```python
from build123d import *

# Parameters (mm, degrees)
SKETCH002_R     = 6
SKETCH002_R_2   = 3
SKETCH002_R_3   = 1.25
SKETCH002_R_4   = 2
SKETCH002_R_5   = 12
PAD_DEPTH       = 28.575
POCKET_DEPTH    = 16.075
SKETCH_R        = 13.05
POCKET001_DEPTH = 10
SKETCH005_R     = 13.05
POCKET002_DEPTH = 10
SKETCH006_R     = 3
POCKET003_DEPTH = 23
SKETCH007_R     = 5
POCKET004_DEPTH = 6.2


with BuildPart() as part:
    # Sketch002 → Pad (new body)
    with BuildSketch(Plane(origin=(0, 0, 0), x_dir=(1, 0, 0), z_dir=(0, 0, -1))):
        with BuildLine():
            Line((22.5, 0), (-41.5, 0))
            Line((-41.5, 0), (-41.5, 96))
            ThreePointArc((-41.5, 96), (-42.671582, 98.828436), (-45.500026, 100))
            Line((-53.999998, 100), (-45.500026, 100))
            ThreePointArc((-58, 104), (-56.828427, 101.171573), (-53.999998, 100))
            Line((-58, 154), (-58, 104))
            ThreePointArc((-53.999999, 158), (-56.828427, 156.828427), (-58, 154))
            Line((-53.999999, 158), (-4, 158))
            ThreePointArc((0, 154), (-1.171573, 156.828427), (-4, 158))
            Line((0, 154), (0, 104.000001))
            ThreePointArc((0, 104.000001), (1.171573, 101.171574), (4, 100.000001))
            Line((22.5, 100.000001), (4, 100.000001))
            Line((22.5, 100.000001), (22.5, 0))
        make_face()
        with Locations((-29, 129)):
            Circle(SKETCH002_R, mode=Mode.SUBTRACT)
        with Locations((-31, 66.5)):
            Circle(SKETCH002_R_2, mode=Mode.SUBTRACT)
        with Locations((-31, 28.5)):
            Circle(SKETCH002_R_2, mode=Mode.SUBTRACT)
        with Locations((-5.43, 152.57)):
            Circle(SKETCH002_R_3, mode=Mode.SUBTRACT)
        with Locations((-52.57, 152.57)):
            Circle(SKETCH002_R_3, mode=Mode.SUBTRACT)
        with Locations((-52.57, 105.43)):
            Circle(SKETCH002_R_3, mode=Mode.SUBTRACT)
        with Locations((-5.43, 105.43)):
            Circle(SKETCH002_R_3, mode=Mode.SUBTRACT)
        with Locations((18.5, 96.000001)):
            Circle(SKETCH002_R_4, mode=Mode.SUBTRACT)
        with Locations((18.5, 4)):
            Circle(SKETCH002_R_4, mode=Mode.SUBTRACT)
        with Locations((-0.5, 50)):
            Circle(SKETCH002_R_5, mode=Mode.SUBTRACT)
    extrude(amount=PAD_DEPTH)

    # Sketch004 → Pocket (cut)
    with BuildSketch(Plane.XY):
        with BuildLine():
            Line((-45, 0), (24, 0))
            Line((24, 0), (24, -104.00002))
            Line((24, -104.00002), (0, -104.00002))
            ThreePointArc((0, -104.00002), (-1.171559, -101.171587), (-3.99998, -100))
            Line((-3.99998, -100), (-45, -100))
            Line((-45, -100), (-45, 0))
        make_face()
    extrude(amount=-POCKET_DEPTH, mode=Mode.SUBTRACT)

    # Sketch → Pocket001 (cut)
    with BuildSketch(Plane(origin=(0, 0, -28.575), x_dir=(1, 0, 0), z_dir=(0, 0, -1))):
        with Locations((-29, 129)):
            Circle(SKETCH_R)
    extrude(amount=-POCKET001_DEPTH, mode=Mode.SUBTRACT)

    # Sketch005 → Pocket002 (cut)
    with BuildSketch(Plane.XY):
        with Locations((-29, -129)):
            Circle(SKETCH005_R)
    extrude(amount=-POCKET002_DEPTH, mode=Mode.SUBTRACT)

    # Sketch006 → Pocket003 (cut)
    with BuildSketch(Plane(origin=(0, 0, -28.575), x_dir=(1, 0, 0), z_dir=(0, 0, -1))):
        with Locations((-52.57, 152.57)):
            Circle(SKETCH006_R)
        with Locations((-5.43, 152.57)):
            Circle(SKETCH006_R)
        with Locations((-52.57, 105.43)):
            Circle(SKETCH006_R)
        with Locations((-5.43, 105.43)):
            Circle(SKETCH006_R)
    extrude(amount=-POCKET003_DEPTH, mode=Mode.SUBTRACT)

    # Sketch007 → Pocket004 (cut)
    with BuildSketch(Plane.XY.offset(-16.075)):
        with Locations((-31, -28.5)):
            Circle(SKETCH007_R)
        with Locations((-31, -66.5)):
            Circle(SKETCH007_R)
        with BuildLine():
            Line((14.5, 0), (22.5, 0))
            Line((22.5, 0), (22.5, -8))
            Line((18.500001, -8), (22.5, -8))
            ThreePointArc((14.5, -4), (15.671573, -6.828428), (18.500001, -8))
            Line((14.5, 0), (14.5, -4))
        make_face()
        with BuildLine():
            Line((22.5, -92.01), (22.5, -100.01))
            Line((22.5, -100.01), (14.5, -100.01))
            Line((14.5, -96.01), (14.5, -100.01))
            ThreePointArc((18.499999, -92.01), (15.671573, -93.181573), (14.5, -96.01))
            Line((18.499999, -92.01), (22.5, -92.01))
        make_face()
    extrude(amount=-POCKET004_DEPTH, mode=Mode.SUBTRACT)


solid = part.part
```
The model under review builds one solid part; all positions refer to its coordinate system, in mm. A direction names the side the tool comes from. Round coordinates to 2 decimals unless told otherwise and drop trailing zeros. Order: outer loops, then holes, each group sorted by start corner. A loop starts at its lowest first (then second) coordinate and runs counter-clockwise, first axis right, second up. Notation, with made-up numbers: (68, -35.75) -> (120, -35.75) arc R24 cw to (120, -15.75) -> close; hole circle Ø5 at (76, 36). An arc over 180 degrees is marked (long way). Use a Markdown table: item, result.
Q1. We need section B-B on z = -13. State how many separate pieces and enclosed holes the cut face has, then the cut area to 3 significant figures.
Values:
| item | result |
|---|---|
| separate pieces | 1 |
| enclosed holes | 5 |
| area | 3,120 mm^2 |
Q2. For line 1 (X direction, y = -105.43, z = -3.1); line 2 (Y direction, x = -5.43, z = -3.55); line 3 (Y direction, x = -52.57, z = -15.5), list the stretches that pass through material, from the lowest coordinate up.
Values:
| item | result |
|---|---|
| line 1 | x = -58 to -53.82, -51.32 to -6.68, -4.18 to 0 |
| line 2 | y = -158 to -153.82, -151.32 to -106.68, -104.18 to -100 |
| line 3 | y = -158 to -155.57, -149.57 to -108.43, -102.43 to -100 |
Q3. Mouldability with a two-part tool opening along X and no side actions: class faces 5 (the cylindrical face through (-43.17, -99.25, -20.44)), 6 (the flat face through (-29, -69, -22.275)), 7 (the flat face through (20, -8, -19)) as +X half, -X half, draft (parallel to the pull), parting line (faces both ways), or undercut.
Values:
| item | result |
|---|---|
| face 5 | -X half |
| face 6 | undercut |
| face 7 | draft |
Q4. Clearance check with flat-ended pins moving along their axes: P1, Ø3, axis at y = -97, z = -20, coming from the +X side; P2, Ø2, axis at x = -44.5, z = -21, coming from the +Y side; P3, Ø11, axis at x = -32, y = -30.5, coming from the +Z side (3 decimals). State where each tip first meets the part, or that it passes through.
Values:
| item | result |
|---|---|
| P1 | stops at x = 14.53 |
| P2 | stops at y = -99.46 |
| P3 | stops at z = -16.075 |
Q5. We need section A-A on y = -50. Write out the cut boundary in (x, z) (3 decimals), then the cut area to 3 significant figures.
Values:
| item | result |
|---|---|
| outline | (-41.5, -28.575) -> (-12.5, -28.575) -> (-12.5, -16.075) -> (-41.5, -16.075) -> close; (11.5, -28.575) -> (22.5, -28.575) -> (22.5, -16.075) -> (11.5, -16.075) -> close |
| area | 500 mm^2 |
Q6. Tool access review of faces 1 (the cylindrical face through (-30.7, -116.06, -4.93)), 2 (the flat face through (20, -2, -22.275)), 3 (the flat face through (-4, -153, -5.575)), 4 (the flat face through (0, -129, -14)): name each direction out of +Z, -Z, +X, -X, +Y, -Y from which nothing blocks a thin tool from reaching the whole face with its end or side.
Values:
| item | result |
|---|---|
| face 1 | +Z |
| face 2 | +Z, +X, +Y |
| face 3 | -Z |
| face 4 | +Z, -Z, +X, -Y |
Q7. We need section D-D on y = -66.5. Write out the cut boundary in (x, z) (3 decimals), then the cut area to 3 significant figures.
Values:
| item | result |
|---|---|
| outline | (-41.5, -28.575) -> (-34, -28.575) -> (-34, -22.275) -> (-36, -22.275) -> (-36, -16.075) -> (-41.5, -16.075) -> close; (-28, -28.575) -> (22.5, -28.575) -> (22.5, -16.075) -> (-26, -16.075) -> (-26, -22.275) -> (-28, -22.275) -> close |
| area | 700 mm^2 |
